Check sheet for the modelled part. Datum: model origin and axes. Units: mm. A direction names the side the tool comes from. Give positions to 0.01 mm unless a question says otherwise; leave off trailing zeros. Order: outer loops, then holes, each group sorted by start corner. A loop starts at its lowest first (then second) coordinate and runs counter-clockwise, first axis right, second up. Notation, with made-up numbers: M -8.75,-4 L 40.25,-4 A29 ccw 40.25,18 Z; hole C -14,47.25 d8. An arc over 180 degrees is marked long. Answer in a Markdown table with one row per item. Add a question column.
from build123d import *

# Parameters (mm, degrees)
F0_R     = 19.84375
F0_R_2   = 12.7
F1_DEPTH = 0.79375
F0_W     = 73.66
F0_H     = 73.66
F0_R_3   = 1.5875
F2_DEPTH = 1.5875


with BuildPart() as f1:
    # F0 (on Top) → F1 (new body)
    with BuildSketch(Plane.XY):
        Circle(F0_R)
        Circle(F0_R_2, mode=Mode.SUBTRACT)
    extrude(amount=F1_DEPTH)

    # F0 (on Top) → F2 (join)
    with BuildSketch(Plane.XY):
        Rectangle(F0_W, F0_H)
        with Locations((-23.8125, -34.13125)):
            Circle(F0_R_3, mode=Mode.SUBTRACT)
        with Locations((-34.13125, -23.8125)):
            Circle(F0_R_3, mode=Mode.SUBTRACT)
        Circle(F0_R, mode=Mode.SUBTRACT)
        with Locations((23.8125, -34.13125)):
            Circle(F0_R_3, mode=Mode.SUBTRACT)
        with Locations((34.13125, -23.8125)):
            Circle(F0_R_3, mode=Mode.SUBTRACT)
        with Locations((-34.13125, 23.8125)):
            Circle(F0_R_3, mode=Mode.SUBTRACT)
        with Locations((-23.8125, 34.13125)):
            Circle(F0_R_3, mode=Mode.SUBTRACT)
        with Locations((34.13125, 23.8125)):
            Circle(F0_R_3, mode=Mode.SUBTRACT)
        with Locations((23.8125, 34.13125)):
            Circle(F0_R_3, mode=Mode.SUBTRACT)
    extrude(amount=F2_DEPTH)


solid = f1.part
Q1. Cross-section at D-D (y = -17.5). Record the boundary of the cut face in (x, z), and give its area (3 significant figures).
Q2. Cross-section at A-A (x = 0). Record the boundary of the cut face in (y, z).
Q3. Go/stop test with a flat-tipped pin: pin 1 (12 mm diameter, centred on x = 8, y = 7, fed in from +Z). Record where the tip stops, or that it passes through.
Q4. Tool access check on faces 5 (the flat face through (-36.83, -1, 1)), 6 (the cylindrical face through (18.927, 5.961, 1.185)). Record the directions out of +Z, -Z, +X, -X, +Y, -Y that give a thin tool (end or side, any length) a straight path to the whole face; none if there is none.
Q5. Draft check along Y on faces 1 (the flat face through (-1, 36.83, 1)), 2 (the flat face through (36.83, -1, 1)), 3 (the cylindrical face through (-33.4, -25.22, 0.78)), 4 (the flat face through (0, -13, 0.794)). Enter one of: pulls with the +Y half, pulls with the -Y half, needs draft (parallel to the pull), parting line crosses it, or undercut.
Q6. Cross-section at C-C (z = 0.5). State how many separate pieces and enclosed holes the cut face has, and give its area (3 significant figures).
Q7. Thickness scan on probe 1 along X at (y, z) = (17, 1.45); probe 2 along Y at (x, z) = (22.5, 1); probe 3 along Y at (x, z) = (4, 1.3). Record the ranges inside material, lowest first.
Values follow:
| question | item | result |
|---|---|---|
| 1 | outline | M -36.83,0 L 36.83,0 L 36.83,1.59 L 9.36,1.59 L 9.36,0.79 L -9.36,0.79 L -9.36,1.59 L -36.83,1.59 Z |
| 1 | area | 102 mm² |
| 2 | outline | M -36.83,0 L -12.7,0 L -12.7,0.79 L -19.84,0.79 L -19.84,1.59 L -36.83,1.59 Z; M 12.7,0 L 36.83,0 L 36.83,1.59 L 19.84,1.59 L 19.84,0.79 L 12.7,0.79 Z |
| 3 | pin 1 | z = 0.79 |
| 4 | face 5 | +Z, -Z, -X, +Y, -Y |
| 4 | face 6 | +Z |
| 5 | face 1 | pulls with the +Y half |
| 5 | face 2 | needs draft |
| 5 | face 3 | undercut |
| 5 | face 4 | undercut |
| 6 | separate pieces | 1 |
| 6 | enclosed holes | 9 |
| 6 | area | 4,860 mm² |
| 7 | probe 1 | -36.83 to -10.24, 10.24 to 36.83 |
| 7 | probe 2 | -36.83 to -35.02, -33.24 to 33.24, 35.02 to 36.83 |
| 7 | probe 3 | -36.83 to -19.44, 19.44 to 36.83 |
